The model under review builds one solid part; all positions refer to its coordinate system, in mm. Face numbers are marked on the shaded views. Coordinates: 2 decimals unless noted, no trailing zeros. Loops run counter-clockwise (first coordinate to the right, second up) from the corner with the lowest first, then second, coordinate; pieces in that order, holes last. Notation, with made-up numbers: M -29.75,6.5 L -13.75,6.5 A22 cw -13.75,18.5 Z; hole C 66,40 d9. An arc over 180 degrees is marked long. Use one line per item in the form item = value.
```python
from build123d import *

# Parameters (mm, degrees)
CROQUIS1_R              = 17
CROQUIS1_R_2            = 1
CROQUIS1_R_3            = 1.6
SALIENTE_EXTRUIR1_DEPTH = 3
CROQUIS2_R              = 17
CROQUIS2_R_2            = 15
SALIENTE_EXTRUIR2_DEPTH = 7
CROQUIS3_R              = 3
CROQUIS3_R_2            = 1.6
SALIENTE_EXTRUIR3_DEPTH = 6
SALIENTE_EXTRUIR4_DEPTH = 5


with BuildPart() as part:
    # Croquis1 → Saliente-Extruir1 (new body)
    with BuildSketch(Plane(origin=(0, 0, 0), x_dir=(1, 0, 0), z_dir=(0, 1, 0))):
        with Locations(Location((0, 0, 0), (0, 0, 270))):
            Circle(CROQUIS1_R)
        with Locations(Location((0, 0, 0), (0, 0, 270))):
            Circle(CROQUIS1_R_2, mode=Mode.SUBTRACT)
        with Locations(Location((-10, 0, 0), (0, 0, 270))):
            Circle(CROQUIS1_R_3, mode=Mode.SUBTRACT)
        with Locations(Location((10, 0, 0), (0, 0, 270))):
            Circle(CROQUIS1_R_3, mode=Mode.SUBTRACT)
    extrude(amount=SALIENTE_EXTRUIR1_DEPTH)

    # Croquis2 → Saliente-Extruir2 (add)
    with BuildSketch(Plane(origin=(0, 3, 0), x_dir=(1, 0, 0), z_dir=(0, 1, 0))):
        with Locations(Location((0, 0, 0), (0, 0, 270))):
            Circle(CROQUIS2_R)
        with Locations(Location((0, 0, 0), (0, 0, 270))):
            Circle(CROQUIS2_R_2, mode=Mode.SUBTRACT)
    extrude(amount=SALIENTE_EXTRUIR2_DEPTH)

    # Croquis3 → Saliente-Extruir3 (add)
    # profile 1 of 2: a face of its own
    with BuildSketch(Plane(origin=(0, 3, 0), x_dir=(1, 0, 0), z_dir=(0, 1, 0))):
        with Locations(Location((10, 0, 0), (0, 0, 270))):
            Circle(CROQUIS3_R)
        with Locations(Location((10, 0, 0), (0, 0, 270))):
            Circle(CROQUIS3_R_2, mode=Mode.SUBTRACT)
    # profile 2 of 2: a face of its own
    with BuildSketch(Plane(origin=(0, 3, 0), x_dir=(1, 0, 0), z_dir=(0, 1, 0))):
        with Locations(Location((-10, 0, 0), (0, 0, 270))):
            Circle(CROQUIS3_R)
        with Locations(Location((-10, 0, 0), (0, 0, 270))):
            Circle(CROQUIS3_R_2, mode=Mode.SUBTRACT)
    extrude(amount=SALIENTE_EXTRUIR3_DEPTH)

    # Croquis4 → Saliente-Extruir4 (add)
    with BuildSketch(Plane(origin=(0, 3, 0), x_dir=(1, 0, 0), z_dir=(0, 1, 0))):
        with BuildLine():
            Line((1, 0), (2, 0))
            ThreePointArc((2, 0), (0, 2), (-2, 0))
            Line((-2, 0), (-1, 0))
            ThreePointArc((-1, 0), (0, 1), (1, 0))
        make_face()
    extrude(amount=SALIENTE_EXTRUIR4_DEPTH)


solid = part.part
```
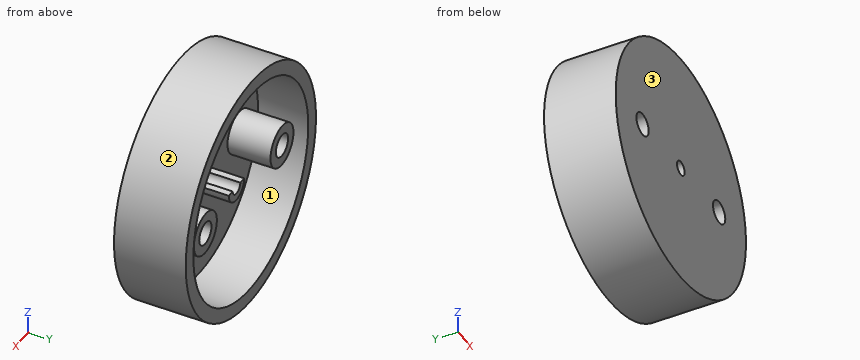
1. Add section C-C (z = 11). State the section outline as (x, y) points, then the cut area to 3 significant figures.
Response values:
outline = M -12.96,0 L 12.96,0 L 12.96,10 L 10.2,10 L 10.2,3 L -10.2,3 L -10.2,10 L -12.96,10 Z
area = 116 mm^2
2. Insertion check: P1, Ø15, axis at x = 4, z = 7, coming from the +Y side; P2, Ø3, axis at x = -10, z = 0, coming from the -Y side (3 decimals); P3, Ø1.1, axis at x = 1.5, y = 6.5, coming from the +Z side; P4, Ø5, axis at x = 10, z = 0, coming from the +Y side. Each pin has a flat end and moves straight along its axis. Give the tip position at first contact, or say it passes through.
Response values:
P1 = 10
P2 = through
P3 = 16.97
P4 = 9
3. Add section B-B (x = 0). State the section outline as (y, z) points, then the cut area to 3 significant figures.
Response values:
outline = M 0,-17 L 10,-17 L 10,-15 L 3,-15 L 3,-2 L 8,-2 L 8,-1 L 0,-1 Z; M 0,1 L 3,1 L 3,15 L 10,15 L 10,17 L 0,17 Z
area = 129 mm^2
4. The part is to be moulded in two halves that separate along X. For the marked faces 1, 2 and 3, say which applies: pulls with the +X half, pulls with the -X half, needs draft (parallel to the pull), parting line crosses it, or undercut.
Response values:
face_1 = undercut
face_2 = parting line crosses it
face_3 = needs draft
5. Wall thickness on line 1 along X through (y, z) = (1.6, 0); line 2 along Z through (x, y) = (-1.5, 3.5); line 3 along Y through (x, z) = (-7, 7.5): over which ranges is each line inside the solid? List them lowest first. Write a range as from..to.
Response values:
line_1 = -17..-11.6, -8.4..-1, 1..8.4, 11.6..17
line_2 = -16.93..-14.92, -1.32..0, 14.92..16.93
line_3 = 0..3
6. Add section D-D (x = 10). State the section outline as (y, z) points, then the cut area to 3 significant figures.
Response values:
outline = M 0,-13.75 L 10,-13.75 L 10,-11.18 L 3,-11.18 L 3,-3 L 9,-3 L 9,-1.6 L 0,-1.6 Z; M 0,1.6 L 9,1.6 L 9,3 L 3,3 L 3,11.18 L 10,11.18 L 10,13.75 L 0,13.75 Z
area = 126 mm^2
7. Add section A-A (y = 3.5). State the section outline as (x, z) points, then the cut area to 3 significant figures.
Response values:
outline = C 0,0 d34; C -10,0 d6; M -2,0 A2 ccw 2,0 L 1,0 A1 cw -1,0 Z; C 10,0 d6; hole C 0,0 d30; hole C -10,0 d3.2; hole C 10,0 d3.2
area = 246 mm^2
